Check sheet for the drawn part. Datum: minimum x, y, z corner. Units: mm. Give positions to 0.01 mm unless a question says otherwise; leave off trailing zeros. Loops run counter-clockwise (first coordinate to the right, second up) from the corner with the lowest first, then second, coordinate; pieces in that order, holes last.
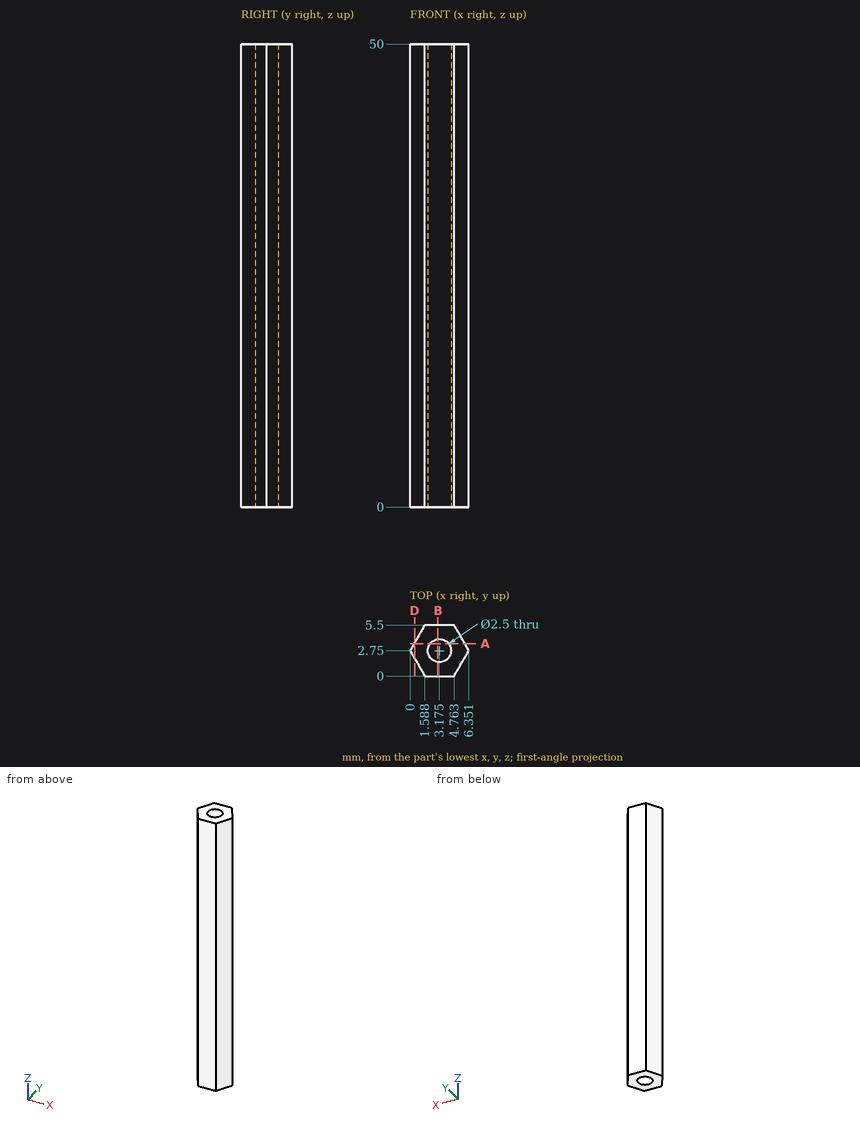
1) Sectioned sample at D-D on x = 0.5. Enter the section's corners in (y, z).
2) Sectioned sample at A-A on y = 3.5. Enter the section's corners in (x, z) (1 decimal), plus the area to 3 significant figures.
3) Scan lines: line 1 along X through (y, z) = (1.65, 24.5) (1 decimal); line 2 along Y through (x, z) = (2.5, 16); line 3 along Y through (x, z) = (3.5, 36). Record each from-to range of solid material in increasing order.
4) Sectioned sample at B-B on x = 3. Enter the section's corners in (y, z), plus the area to 3 significant figures.
5) Depth check by flat-ended pin: P1, Ø1.5, axis at y = 3, z = 21.5, coming from the -X side. Enter the tip coordinate at first touch or a pass-through.
Determined:
1. outline: (1.88, 0) - (3.62, 0) - (3.62, 50) - (1.88, 50) - close
2. outline: (0.4, 0) - (2.2, 0) - (2.2, 50) - (0.4, 50) - close; (4.2, 0) - (5.9, 0) - (5.9, 50) - (4.2, 50) - close
2. area: 174 mm2
3. line 1: x = 0.6 to 2.6, 3.8 to 5.7
3. line 2: y = 0 to 1.7, 3.8 to 5.5
3. line 3: y = 0 to 1.54, 3.96 to 5.5
4. outline: (0, 0) - (1.51, 0) - (1.51, 50) - (0, 50) - close; (3.99, 0) - (5.5, 0) - (5.5, 50) - (3.99, 50) - close
4. area: 151 mm2
5. P1: stops at x = 0
